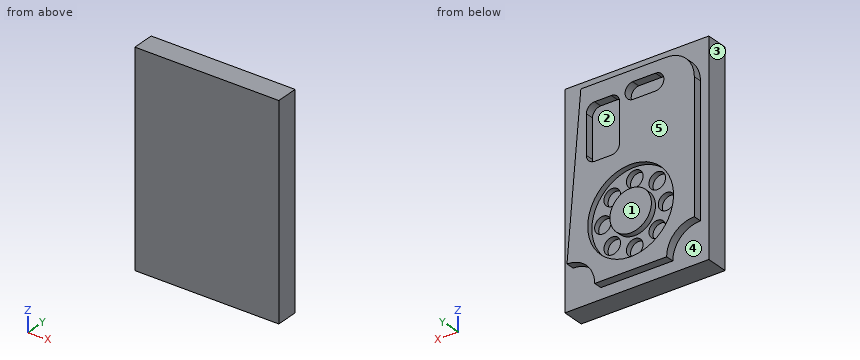
Autodesk Inventor part; units mm, degrees
ref_plane "YZ Plane" through (0, 0, 0) normal (1, 0, 0) x (0, 1, 0)
ref_plane "XZ Plane" through (0, 0, 0) normal (0, 1, 0) x (-1, 0, 0)
ref_plane "XY Plane" through (0, 0, 0) normal (0, 0, 1) x (1, 0, 0)
sketch "Sketch1" plane through (0, 0, 0) normal (0, 1, 0) x (-1, 0, 0)
  line L0 (26, 37.5) -> (-26, 37.5)
  line L1 (-26, 37.5) -> (-26, -37.5)
  line L2 (-26, -37.5) -> (26, -37.5)
  line L3 (26, -37.5) -> (26, 37.5)
  line L4 (26, 37.5) -> (-26, -37.5) construction
  line L5 (-26, 37.5) -> (26, -37.5) construction
  point P0 (0, 0)
  dimension "d0" = 52
  dimension "d1" = 75
extrude "Extrusion1" add sketch "Sketch1" along normal blind 8
sketch "Sketch2" plane through (0, 8, 0) normal (0, 1, 0) x (1, 0, 0)
  arc A0 (-23, 23.5) -> (-13, 33.5) centre (-23, 33.5) ccw
  line L0 (26, 37.5) -> (-26, 37.5)
  line L1 (-26, 37.5) -> (-26, -37.5)
  arc A1 (13, 33.5) -> (23, 23.5) centre (23, 33.5) ccw
  line L2 (26, -37.5) -> (26, 37.5)
  line L3 (-13, 33.5) -> (13, 33.5)
  line L4 (-23, -23.5) -> (-23, 27.9055)
  arc A2 (-23, -23.5) -> (-13, -33.5) centre (-13, -23.5) ccw
  line L5 (-13, -33.5) -> (18, -33.5)
  line L6 (-26, -37.5) -> (26, -37.5)
  line L7 (18, -33.5) -> (23, 23.5)
  line L8 (7, -27.5) -> (13, -27.5)
  line L9 (16, -24.5) -> (16, -10.5)
  line L10 (13, -7.5) -> (7, -7.5)
  line L11 (4, -10.5) -> (4, -24.5)
  line L12 (4, -27.5) -> (16, -7.5) construction
  line L13 (16, -27.5) -> (4, -7.5) construction
  line L14 (-9, -29.5) -> (-0.6728, -29.5)
  line L15 (-0.6728, -23.5) -> (-9, -23.5)
  line L16 (-9, -29.5) -> (-0.6728, -23.5) construction
  line L17 (-0.6728, -29.5) -> (-9, -23.5) construction
  arc A3 (-9, -23.5) -> (-9, -29.5) centre (-9, -26.5) ccw
  arc A4 (-0.6728, -29.5) -> (-0.6728, -23.5) centre (-1, -26.5) ccw
  arc A5 (4, -24.5) -> (7, -27.5) centre (7, -24.5) ccw
  arc A6 (7, -7.5) -> (4, -10.5) centre (7, -10.5) ccw
  arc A7 (16, -10.5) -> (13, -7.5) centre (13, -10.5) ccw
  arc A8 (13, -27.5) -> (16, -24.5) centre (13, -24.5) ccw
  point P0 (0, 0)
  point P1 (10, -17.5)
  point P2 (-4.8364, -26.5)
  dimension "d4" = 20
  dimension "d5" = 4
  dimension "d6" = 3
  dimension "d7" = 4
  dimension "d8" = 3
  dimension "d9" = 20
  dimension "d10" = 3
  dimension "d14" = 3
  dimension "d15" = 4
  dimension "d18" = 8
  dimension "d19" = 16
  dimension "d20" = 22
  dimension "d22" = 4
  dimension "d23" = 20
  dimension "d24" = 30
  dimension "d25" = 10
  dimension "d26" = 6
  dimension "d27" = 6
  dimension "d29" = 11
  dimension "d30" = 27
  dimension "d31" = 35
  dimension "d32" = 49
  dimension "d33" = 52
  dimension "d38" = 3
extrude "Extrusion2" add sketch "Sketch2" along normal blind 3 contours A0 L3 A1 L7 L5 A2 L4
sketch "Sketch3" plane through (0, 11, 0) normal (0, 1, 0) x (1, 0, 0)
  circle A0 centre (0, 13.5) radius 15.5
  circle A1 centre (0, 13.5) radius 7.5
  line L0 (-26, -37.5) -> (26, -37.5)
  line L1 (26, -37.5) -> (26, 37.5)
  point P0 (0, 0)
  dimension "d41" = 15
  dimension "d42" = 31
  dimension "d43" = 51
  dimension "d44" = 26
extrude "Extrusion3" cut sketch "Sketch3" against normal blind 2
sketch "Sketch4" plane through (0, 9, -13.5) normal (0, 1, 0) x (1, 0, 0)
  circle A0 centre (0, 0) radius 7.5
  circle A1 centre (0, 0) radius 11.5
  circle A2 centre (11.5, 0) radius 3
  circle A3 centre (8.1317, 8.1317) radius 3
  circle A4 centre (0, 11.5) radius 3
  circle A5 centre (-8.1317, 8.1317) radius 3
  circle A6 centre (-11.5, 0) radius 3
  circle A7 centre (-8.1317, -8.1317) radius 3
  circle A8 centre (0, -11.5) radius 3
  circle A9 centre (8.1317, -8.1317) radius 3
  point P0 (0, -13.5)
  dimension "d47" = 23
  dimension "d48" = 6
  dimension "d51" = 360
extrude "Extrusion4" cut sketch "Sketch4" against normal blind 2 contours A1 A2 | A1 A2 | A3 A1 | A1 A3 | A9 A1 | A1 A9 | A4 A1 | A1 A4 | A8 A1 | A1 A8 | A5 A1 | A1 A5 | A7 A1 | A1 A7 | A6 A1 | A1 A6
properties part number "Exercise2"
Verification items for the finished model (mm, model axes). Face numbers are marked on the shaded views. A direction names the side the tool comes from. Coordinates: 2 decimals unless noted, no trailing zeros. Order: outer loops, then holes, each group sorted by start corner. A loop starts at its lowest first (then second) coordinate and runs counter-clockwise, first axis right, second up. Notation, with made-up numbers: M 57,31 L 67,31 A24 ccw 67,62 Z; hole C 85,-4 d8. An arc over 180 degrees is marked long. Return JSON: item names as keys, results as strings.
1) Cross-section at B-B, the plane z = -31. Record the boundary of the cut face in (x, y).
Answer list:
{"outline": "M -26,0 L 26,0 L 26,8 L 13.32,8 L 13.32,11 L -13.32,11 L -13.32,8 L -26,8 Z"}
2) Access from +Z, -Z, +X, -X, +Y, -Y to the whole of each face (thin tool, end or side, straight path). Record for the marked faces 4 and 5.
Answer list:
{"face 4": "+Y", "face 5": "+Z, -Z, +X, -X, +Y"}
3) Thickness scan on L1, parallel to X at y = 7.8, z = -13.5; L2, parallel to X at y = 10.15, z = -13.5; L3, parallel to Y at x = 8.5, z = 19.5. Record the ranges inside material, lowest first. Write a range as [from, to].
Answer list:
{"L1": "[-26, -14.5], [-8.5, 8.5], [14.5, 26]", "L2": "[-23, -15.5], [-7.5, 7.5], [15.5, 22.12]", "L3": "[0, 8]"}
4) Cross-section at A-A, the plane x = 12. Record the boundary of the cut face in (y, z).
Answer list:
{"outline": "M 0,-37.5 L 8,-37.5 L 8,-33.5 L 11,-33.5 L 11,-23.31 L 9,-23.31 L 9,-16.46 L 7,-16.46 L 7,-10.54 L 9,-10.54 L 9,-3.69 L 11,-3.69 L 11,7.5 L 8,7.5 L 8,27.5 L 11,27.5 L 11,33.5 L 8,33.5 L 8,37.5 L 0,37.5 Z"}
5) Release check for a two-part mould opening along X. For the marked faces 1, 2 and 3 record: +X half, -X half, draft (parallel to the pull), parting line (faces both ways), or undercut.
Answer list:
{"face 1": "draft", "face 2": "undercut", "face 3": "-X half"}
6) Gauge pin test, flat ends, axial feed: pin 1 (3.5 mm diameter, centred on x = -11.5, z = -13.5, fed in from +Y); pin 2 (2.5 mm diameter, centred on x = 7.5, y = 10, fed in from +Z); pin 3 (6.5 mm diameter, centred on x = -12, z = -14.5, fed in from +Y); pin 4 (3.5 mm diameter, centred on y = 9.5, z = 5.5, fed in from -X). Record the tip position at first contact, or that the pin passes through.
Answer list:
{"pin 1": "y = 7", "pin 2": "z = 33.5", "pin 3": "y = 9", "pin 4": "x = -26"}
7) Cross-section at C-C, the plane z = 26.5. Record the boundary of the cut face in (x, y), and give its area (3 significant figures).
Answer list:
{"outline": "M -26,0 L 26,0 L 26,8 L 18.61,8 L 18.61,11 L 15.24,11 L 15.24,8 L 4.76,8 L 4.76,11 L 2.02,11 L 2.02,8 L -12,8 L -12,11 L -22.54,11 L -22.54,8 L -26,8 Z", "area": "466 mm2"}
